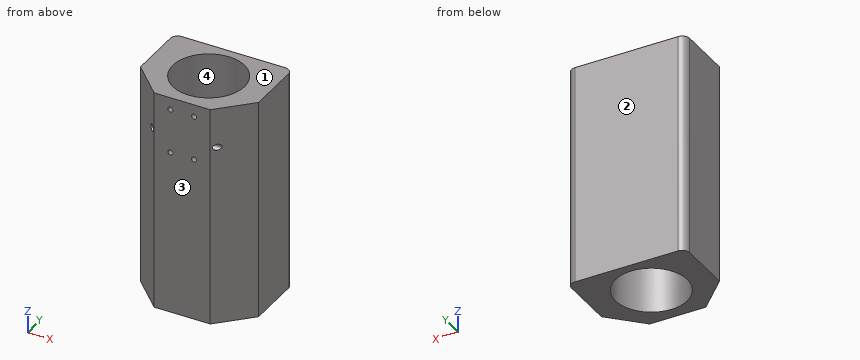
from build123d import *

# Parameters (mm, degrees)
SKETCH1_W               = 80
SKETCH1_H               = 60
SKETCH1_R               = 24.25
BOSS_EXTRUDE1_DEPTH     = 150
SKETCH2_W               = 80
SKETCH2_H               = 150
BOSS_EXTRUDE2_DEPTH     = 2
CUT_EXTRUDE1_DEPTH      = 159.505520409
SKETCH4_R               = 2.1
CUT_EXTRUDE2_DEPTH      = 24
CUT_EXTRUDE3_START      = -24
SKETCH5_R               = 2.1
CUT_EXTRUDE3_DEPTH      = 24
CUT_EXTRUDE4_REACH      = 169.165
CUT_EXTRUDE4_END_RADIUS = 24.25
SKETCH6_R               = 1.75
FILLET1_R               = 5


with BuildPart() as part:
    # Sketch1 → Boss-Extrude1 (new body)
    with BuildSketch(Plane.XY):
        Rectangle(SKETCH1_W, SKETCH1_H)
        Circle(SKETCH1_R, mode=Mode.SUBTRACT)
    extrude(amount=BOSS_EXTRUDE1_DEPTH)

    # Sketch2 → Boss-Extrude2 (add)
    with BuildSketch(Plane.XZ.offset(30)):
        with Locations((0, 75)):
            Rectangle(SKETCH2_W, SKETCH2_H)
    extrude(amount=BOSS_EXTRUDE2_DEPTH)

    # Sketch3 → Cut-Extrude1 (cut, through all)
    with BuildSketch(Plane.XY.offset(150)):
        Polygon((-40, -11), (-40, -32), (-19, -32), align=None)
        Polygon((19, -32), (40, -11), (40, -32), align=None)
    extrude(amount=-CUT_EXTRUDE1_DEPTH, mode=Mode.SUBTRACT)

    # Sketch4 → Cut-Extrude2 (cut)
    with BuildSketch(Plane(origin=(40, 0, 0), x_dir=(0, 0, -1), z_dir=(1, 0, 0))):
        with Locations(Location((-123, -29, 0), (0, 0, 90))):
            Circle(SKETCH4_R)
    extrude(amount=-CUT_EXTRUDE2_DEPTH, mode=Mode.SUBTRACT)

    # Sketch5 → Cut-Extrude3 (cut)
    with BuildSketch(Plane.ZY.offset(40).offset(CUT_EXTRUDE3_START)):
        with Locations(Location((123, -29, 0), (0, 0, 90))):
            Circle(SKETCH5_R)
    extrude(amount=CUT_EXTRUDE3_DEPTH, mode=Mode.SUBTRACT)

    # Cut-Extrude4: up to this cylinder (the profile starts outside it)
    cut_extrude4_end = Plane(origin=(0, 0, 126.7), z_dir=(0, 0, -1)) * Cylinder(CUT_EXTRUDE4_END_RADIUS, 417.83, mode=Mode.PRIVATE)
    # Sketch6 → Cut-Extrude4 (cut, up to the surface)
    with BuildSketch(Plane.XZ.offset(32), mode=Mode.PRIVATE) as cut_extrude4_sk1:
        with Locations(Location((-8, 141.7, 0), (0, 0, 270))):
            Circle(SKETCH6_R)
    cut_extrude4_tool1 = extrude(cut_extrude4_sk1.sketch, amount=-CUT_EXTRUDE4_REACH, mode=Mode.PRIVATE) - cut_extrude4_end
    add(cut_extrude4_tool1.solids().sort_by_distance((-8, -32, 141.7))[0], mode=Mode.SUBTRACT)
    # Sketch6 → Cut-Extrude4 (cut, up to the surface)
    with BuildSketch(Plane.XZ.offset(32), mode=Mode.PRIVATE) as cut_extrude4_sk2:
        with Locations(Location((-8, 111.7, 0), (0, 0, 270))):
            Circle(SKETCH6_R)
    cut_extrude4_tool2 = extrude(cut_extrude4_sk2.sketch, amount=-CUT_EXTRUDE4_REACH, mode=Mode.PRIVATE) - cut_extrude4_end
    add(cut_extrude4_tool2.solids().sort_by_distance((-8, -32, 111.7))[0], mode=Mode.SUBTRACT)
    # Sketch6 → Cut-Extrude4 (cut, up to the surface)
    with BuildSketch(Plane.XZ.offset(32), mode=Mode.PRIVATE) as cut_extrude4_sk3:
        with Locations(Location((8, 111.7, 0), (0, 0, 270))):
            Circle(SKETCH6_R)
    cut_extrude4_tool3 = extrude(cut_extrude4_sk3.sketch, amount=-CUT_EXTRUDE4_REACH, mode=Mode.PRIVATE) - cut_extrude4_end
    add(cut_extrude4_tool3.solids().sort_by_distance((8, -32, 111.7))[0], mode=Mode.SUBTRACT)
    # Sketch6 → Cut-Extrude4 (cut, up to the surface)
    with BuildSketch(Plane.XZ.offset(32), mode=Mode.PRIVATE) as cut_extrude4_sk4:
        with Locations(Location((8, 141.7, 0), (0, 0, 270))):
            Circle(SKETCH6_R)
    cut_extrude4_tool4 = extrude(cut_extrude4_sk4.sketch, amount=-CUT_EXTRUDE4_REACH, mode=Mode.PRIVATE) - cut_extrude4_end
    add(cut_extrude4_tool4.solids().sort_by_distance((8, -32, 141.7))[0], mode=Mode.SUBTRACT)

    # Fillet1
    fillet1_edges = [part.edges().sort_by_distance(p)[0] for p in [
        (-40, 30, 75),
        (40, 30, 75),
    ]]
    fillet(fillet1_edges, radius=FILLET1_R)


solid = part.part
Read the model definition and answer for the solid it produces. Units are mm, in the model's axes. Face numbers are marked on the shaded views. Give positions to 0.01 mm unless a question says otherwise; leave off trailing zeros. Write each loop counter-clockwise with the first axis right and the second up, starting at its lowest first coordinate (ties: lowest second). Pieces come first, ordered by that corner, then holes. Notation, with made-up numbers: (1, -37.5) - (22, -37.5) arc R27 cw to (22, 1.5) - close; hole circle Ø1 at (84, -23). An arc over 180 degrees is marked (long way). Answer in a Markdown table with one row per item. Add a question column.
Item 1: Determine the mould class of the marked faces 1, 2, 3 and 4 for opening direction Y: pulls with the +Y half, pulls with the -Y half, needs draft (parallel to the pull), parting line crosses it, or undercut.
Item 2: Section C-C, the plane y = 22.5 is taken. Write down the section's boundary in (x, z).
Item 3: Section B-B, the plane z = 123 is taken. Write down the section's boundary in (x, y), and give its area (3 significant figures).
Item 4: Section A-A, the plane x = 0 is taken. Write down the section's boundary in (y, z), and give its area (4 significant figures).
Item 5: Find the intervals of material crossed by L1, parallel to Z at x = 8, y = -24; L2, parallel to X at y = -25, z = 111; L3, parallel to X at y = -29, z = 141, in increasing order.
Item 6: Section D-D, the plane x = -8 is taken. Write down the section's boundary in (y, z), and give its area (3 significant figures).
Item 7: Flat-ended cylindrical pins translate along their axes: P1, Ø4.5, axis at y = -30, z = 123.5, coming from the -X side; P2, Ø2.5, axis at y = -29, z = 123, coming from the -X side; P3, Ø4, axis at y = -29, z = 123, coming from the +X side. Find the tip coordinate at first contact, or state that the pin passes through.
Recorded:
| question | item | result |
|---|---|---|
| 1 | face 1 | needs draft |
| 1 | face 2 | pulls with the +Y half |
| 1 | face 3 | pulls with the -Y half |
| 1 | face 4 | undercut |
| 2 | outline | (-40, 0) - (-9.05, 0) - (-9.05, 150) - (-40, 150) - close; (9.05, 0) - (40, 0) - (40, 150) - (9.05, 150) - close |
| 3 | outline | (-40, -11) - (-24.1, -26.9) - (-16, -26.9) - (-16, -31.1) - (-19.9, -31.1) - (-19, -32) - (19, -32) - (19.9, -31.1) - (16, -31.1) - (16, -26.9) - (24.1, -26.9) - (40, -11) - (40, 25) arc R5 ccw to (35, 30) - (-35, 30) arc R5 ccw to (-40, 25) - close; hole circle Ø48.5 at (0, 0) |
| 3 | area | 2,610 mm2 |
| 4 | outline | (-32, 0) - (-24.25, 0) - (-24.25, 150) - (-32, 150) - close; (24.25, 0) - (30, 0) - (30, 150) - (24.25, 150) - close |
| 4 | area | 2,025 mm2 |
| 5 | L1 | z = 0 to 109.95, 113.45 to 139.95, 143.45 to 150 |
| 5 | L2 | x = -26 to -9.6, -6.4 to 6.4, 9.6 to 26 |
| 5 | L3 | x = -22 to -9.6, -6.4 to 6.4, 9.6 to 22 |
| 6 | outline | (-32, 0) - (-22.89, 0) - (-22.89, 109.95) - (-32, 109.95) - close; (-32, 113.45) - (-22.89, 113.45) - (-22.89, 139.95) - (-32, 139.95) - close; (-32, 143.45) - (-22.89, 143.45) - (-22.89, 150) - (-32, 150) - close; (22.89, 0) - (30, 0) - (30, 150) - (22.89, 150) - close |
| 6 | area | 2,370 mm2 |
| 7 | P1 | stops at x = -22.69 |
| 7 | P2 | stops at x = -16 |
| 7 | P3 | stops at x = 16 |
